Check sheet for the modelled part. Datum: model origin and axes. Units: mm. Round coordinates to 2 decimals unless told otherwise and drop trailing zeros. Write each loop counter-clockwise with the first axis right and the second up, starting at its lowest first coordinate (ties: lowest second). Pieces come first, ordered by that corner, then holes.
Item 1: Go/stop test with a flat-tipped pin: pin 1 Ø2 at (x, y) = (4, 2.5) entering from +Z. Record where the tip stops, or that it passes through.
Item 2: Cross-section at B-B on x = -36. Enter the section's corners in (y, z).
Item 3: Cross-section at A-A on z = 54. Enter the section's corners in (x, y).
Item 4: Material ranges on line 1 (X direction, y = 3.5, z = -37.5); line 2 (Z direction, x = -23, y = 1.25); line 3 (X direction, y = 3.5, z = -2), recorded low to high.
Item 5: Cross-section at C-C on y = 1. Count the separate pieces of the cut face and the enclosed holes in it, plus the area to 3 significant figures.
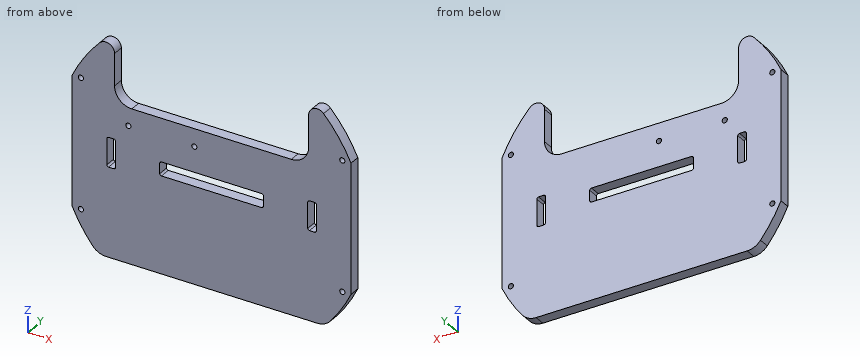
from build123d import *

# Parameters (mm, degrees)
MAIN_BODY_DEPTH    = 6.35
SKETCH6_R          = 1.524
FRONT_IR_DEPTH     = 121.168600308
SKETCH10_W         = 38.1
SKETCH10_H         = 25.908
GRABBER_SLOT_DEPTH = 121.168600308
SKETCH11_W         = 5
SKETCH11_H         = 17
SKETCH11_W_2       = 60
SKETCH11_H_2       = 8
WIRE_SLOTS_DEPTH   = 121.168600308
SKETCH13_R         = 1.5
F_2ND_LEVEL_DEPTH  = 121.168600308
CUT_EXTRUDE1_DEPTH = 121.168600308
FILLET1_R          = 5
FILLET2_R          = 10
CUT_EXTRUDE2_START = -10
CUT_EXTRUDE2_DEPTH = 10
FILLET3_R          = 10
FILLET4_R          = 1
SKETCH17_R         = 1.5
CUT_EXTRUDE3_DEPTH = 103.170168296


with BuildPart() as part:
    # Sketch1 → Main Body (new body)
    with BuildSketch(Plane(origin=(0, 0, 0), x_dir=(1, 0, 0), z_dir=(0, 1, 0))):
        with BuildLine():
            Line((-80.603721998, 37.5), (-80.603721998, -37.5))
            ThreePointArc((-80.603721998, -37.5), (0, -88.9), (80.603721998, -37.5))
            Line((80.603721998, -37.5), (80.603721998, 37.5))
            ThreePointArc((80.603721998, 37.5), (0, 88.9), (-80.603721998, 37.5))
        make_face()
    extrude(amount=MAIN_BODY_DEPTH)

    # Sketch6 → Front IR (cut, through all)
    with BuildSketch(Plane(origin=(0, 6.35, 0), x_dir=(1, 0, 0), z_dir=(0, 1, 0))):
        with Locations(Location((-12.7, -69.596, 0), (0, 0, 270))):
            Circle(SKETCH6_R)
        with Locations(Location((12.7, -69.596, 0), (0, 0, 270))):
            Circle(SKETCH6_R)
    extrude(amount=-FRONT_IR_DEPTH, mode=Mode.SUBTRACT)

    # Sketch10 → Grabber slot (cut, through all)
    with BuildSketch(Plane(origin=(0, 6.35, 0), x_dir=(1, 0, 0), z_dir=(0, 1, 0))):
        with Locations((0, -88.9)):
            Rectangle(SKETCH10_W, SKETCH10_H)
    extrude(amount=-GRABBER_SLOT_DEPTH, mode=Mode.SUBTRACT)

    # Sketch11 → Wire slots (cut, through all)
    with BuildSketch(Plane(origin=(0, 6.35, 0), x_dir=(1, 0, 0), z_dir=(0, 1, 0))):
        with Locations((-58.103721998, 0)):
            Rectangle(SKETCH11_W, SKETCH11_H)
        Rectangle(SKETCH11_W_2, SKETCH11_H_2)
        with Locations((58.103721998, 0)):
            Rectangle(SKETCH11_W, SKETCH11_H)
    extrude(amount=-WIRE_SLOTS_DEPTH, mode=Mode.SUBTRACT)

    # Sketch13 → 2nd level (cut, through all)
    with BuildSketch(Plane(origin=(0, 6.35, 0), x_dir=(1, 0, 0), z_dir=(0, 1, 0))):
        with Locations(Location((75.603721998, -37.5, 0), (0, 0, 270))):
            Circle(SKETCH13_R)
        with Locations(Location((-75.603721998, -37.5, 0), (0, 0, 270))):
            Circle(SKETCH13_R)
        with Locations(Location((75.603721998, 37.5, 0), (0, 0, 270))):
            Circle(SKETCH13_R)
        with Locations(Location((-75.603721998, 37.5, 0), (0, 0, 270))):
            Circle(SKETCH13_R)
    extrude(amount=-F_2ND_LEVEL_DEPTH, mode=Mode.SUBTRACT)

    # Sketch14 → Cut-Extrude1 (cut, through all)
    with BuildSketch(Plane(origin=(0, 6.35, 0), x_dir=(1, 0, 0), z_dir=(0, 1, 0))):
        with BuildLine():
            Line((56.134, -68.93608666), (56.134, -28.93608666))
            Line((56.134, -28.93608666), (-56.134, -28.93608666))
            Line((-56.134, -28.93608666), (-56.134, -68.93608666))
            ThreePointArc((-56.134, -68.93608666), (-38.642602624, -80.062221194), (-19.05, -86.834944003))
            Line((-19.05, -86.834944003), (-19.05, -75.946))
            Line((-19.05, -75.946), (19.05, -75.946))
            Line((19.05, -75.946), (19.05, -86.834944003))
            ThreePointArc((19.05, -86.834944003), (38.642602624, -80.062221194), (56.134, -68.93608666))
        make_face()
    extrude(amount=-CUT_EXTRUDE1_DEPTH, mode=Mode.SUBTRACT)

    # Fillet1
    fillet1_edges = [part.edges().sort_by_distance(p)[0] for p in [
        (56.134, 3.175, 68.93608666),
        (-56.134, 3.175, 68.93608666),
    ]]
    fillet(fillet1_edges, radius=FILLET1_R)

    # Fillet2
    fillet2_edges = [part.edges().sort_by_distance(p)[0] for p in [
        (-56.134, 3.175, 28.93608666),
        (56.134, 3.175, 28.93608666),
    ]]
    fillet(fillet2_edges, radius=FILLET2_R)

    # Sketch16 → Cut-Extrude2 (cut)
    with BuildSketch(Plane(origin=(0, 6.35, 0), x_dir=(1, 0, 0), z_dir=(0, 1, 0)).offset(CUT_EXTRUDE2_START)):
        with BuildLine():
            Line((65.598856697, 60), (-65.598856697, 60))
            ThreePointArc((-65.598856697, 60), (0, 88.9), (65.598856697, 60))
        make_face()
    extrude(amount=CUT_EXTRUDE2_DEPTH, mode=Mode.SUBTRACT)

    # Fillet3
    fillet3_edges = [part.edges().sort_by_distance(p)[0] for p in [
        (-65.598856697, 3.175, -60),
        (65.598856697, 3.175, -60),
    ]]
    fillet(fillet3_edges, radius=FILLET3_R)

    # Fillet4
    fillet4_edges = [part.edges().sort_by_distance(p)[0] for p in [
        (-30, 3.175, 4),
        (-30, 3.175, -4),
        (30, 3.175, -4),
        (30, 3.175, 4),
        (55.603721998, 3.175, 8.5),
        (55.603721998, 3.175, -8.5),
        (60.603721998, 3.175, -8.5),
        (60.603721998, 3.175, 8.5),
        (-60.603721998, 3.175, 8.5),
        (-60.603721998, 3.175, -8.5),
        (-55.603721998, 3.175, -8.5),
        (-55.603721998, 3.175, 8.5),
    ]]
    fillet(fillet4_edges, radius=FILLET4_R)

    # Sketch17 → Cut-Extrude3 (cut, through all)
    with BuildSketch(Plane(origin=(0, 6.35, 0), x_dir=(1, 0, 0), z_dir=(0, 1, 0))):
        with Locations(Location((-48.1, -18.678710205, 0), (0, 0, 270))):
            Circle(SKETCH17_R)
        with Locations(Location((-10, -18.678710205, 0), (0, 0, 270))):
            Circle(SKETCH17_R)
    extrude(amount=-CUT_EXTRUDE3_DEPTH, mode=Mode.SUBTRACT)


solid = part.part
Response values:
1. pin 1: stops at z = 28.94
2. outline: (0, -60) - (6.35, -60) - (6.35, 28.94) - (0, 28.94) - close
3. outline: (-70.62, 0) - (-56.13, 0) - (-56.13, 6.35) - (-70.62, 6.35) - close; (56.13, 0) - (70.62, 0) - (70.62, 6.35) - (56.13, 6.35) - close
4. line 1: x = -80.6 to -77.1, -74.1 to 74.1, 77.1 to 80.6
4. line 2: z = -60 to -4, 4 to 28.94
4. line 3: x = -80.6 to -60.6, -55.6 to -30, 30 to 55.6, 60.6 to 80.6
5. separate pieces: 1
5. enclosed holes: 9
5. area: 14,600 mm2
